```python
from build123d import *

# Parameters (mm, degrees)
FILLET2_SIZE = 0.5


with BuildPart() as part:
    # Sketch1 → Revolve1 (revolve)
    with BuildSketch(Plane.XY, mode=Mode.PRIVATE) as revolve1_sk:
        Polygon((0, 5), (3.5, 5), (6, 0), (2.75, 0), (2.75, 4), (0, 4), align=None)
    revolve(revolve1_sk.sketch.rotate(Axis((0, 0, 0), (0, 1, 0)), 90), axis=Axis((0, 0, 0), (0, 1, 0)))

    # Fillet1
    # a fillet whose section is not a circle: 0.5 mm, written as the material it takes off along each edge
    with BuildSketch(Plane(origin=(0, 5, 0), x_dir=(0, 0, -1), z_dir=(1, 0, 0))) as fillet1_piece_1:
        with BuildLine():
            add(Edge.make_bspline([(3.190983006, 0), (3.246118173, 0), (3.30125334, 0), (3.424221159, -0.01541979), (3.520097448, -0.074674596), (3.588882209, -0.177764417), (3.613539405, -0.22707881), (3.638196601, -0.276393202)], knots=[0, 0, 0, 0, 0, 0, 0.5, 0.5, 1, 1, 1, 1, 1, 1], degree=5))
            Line((3.638196601, -0.276393202), (3.5, 0))
            Line((3.5, 0), (3.190983006, 0))
        make_face()
    revolve(axis=Axis((0, 5, 0), (0, 1, 0)), mode=Mode.SUBTRACT)

    # Fillet2
    # a fillet whose section is not a circle: 0.5 mm, written as the material it takes off along each edge
    with BuildSketch(Plane(origin=(0, 0, 0), x_dir=(0, 0, -1), z_dir=(1, 0, 0))) as fillet2_piece_1:
        with BuildLine():
            add(Edge.make_bspline([(2.75 + FILLET2_SIZE, 0), (2.75 + FILLET2_SIZE * 0.831801948466, 0), (2.75 + FILLET2_SIZE * 0.663603896932, 0), (2.75 + FILLET2_SIZE * 0.292893218813, FILLET2_SIZE * 0.0716919198361), (2.75 + FILLET2_SIZE * 0.0716919198361, FILLET2_SIZE * 0.292893218813), (2.75, FILLET2_SIZE * 0.663603896932), (2.75, FILLET2_SIZE * 0.831801948466), (2.75, FILLET2_SIZE)], knots=[0, 0, 0, 0, 0, 0, 0.5, 0.5, 1, 1, 1, 1, 1, 1], degree=5))
            Line((2.75, FILLET2_SIZE), (2.75, 0))
            Line((2.75, 0), (2.75 + FILLET2_SIZE, 0))
        make_face()
    revolve(axis=Axis((0, 0, 0), (0, 1, 0)), mode=Mode.SUBTRACT)


solid = part.part
```
Input: part model. Units: mm. Frame: model coordinates. A direction names the side the tool comes from. Round coordinates to 2 decimals unless told otherwise and drop trailing zeros. Loops run counter-clockwise (first coordinate to the right, second up) from the corner with the lowest first, then second, coordinate; pieces in that order, holes last. Notation, with made-up numbers: M 70.5,36.25 L 104.5,36.25 A13 ccw 104.5,47.25 Z; hole C 41,83.5 d2. An arc over 180 degrees is marked long. Answer in a Markdown table with one row per item. Add a question column.
1. Section A-A (y = 1.8). Output: boundary loops of the cut face in (x, z), and give its area (3 significant figures).
2. Ray query, probe 1 along Z at (x, y) = (-2.25, 2.2); probe 2 along X at (y, z) = (2, 0.75); probe 3 along X at (y, z) = (1.5, 0). Return the intervals inside material, ascending.
3. Mould query, pull axis X, two halves, no side actions, for faces 3 (the face through (0, 5, 0)), 4 (the face through (-1.14, 4.43, -3.61)), 5 (the face through (0, 4, 0)). Classes: released by +X, released by -X, zero draft, split by the parting line, or undercut.
4. Contact query for flat-ended pins moving along their axis: pin 1 (3 mm diameter, centred on x = 3.5, y = 2, fed in from +Z); pin 2 (1 mm diameter, centred on y = 2, z = 0, fed in from -X); pin 3 (1 mm diameter, centred on y = 4, z = -0.5, fed in from -X). Output: stop coordinate, or through.
5. Set-up query: faces 1 (the face through (3, 0, -3)), 2 (the face through (2.685, 2.274, 0.596)). Return all of +Z, -Z, +X, -X, +Y, -Y with unobstructed straight access to the full face (end or side cutting, diameter ignored); none if empty.
6. Section B-B (y = 3.7). Output: boundary loops of the cut face in (x, z), and give its area (3 significant figures).
Values follow:
| question | item | result |
|---|---|---|
| 1 | outline | C 0,0 d10.2; hole C 0,0 d5.5 |
| 1 | area | 58.0 mm^2 |
| 2 | probe 1 | -4.35 to -1.58, 1.58 to 4.35 |
| 2 | probe 2 | -4.94 to -2.65, 2.65 to 4.94 |
| 2 | probe 3 | -5.25 to -2.75, 2.75 to 5.25 |
| 3 | face 3 | zero draft |
| 3 | face 4 | split by the parting line |
| 3 | face 5 | undercut |
| 4 | pin 1 | z = 4.97 |
| 4 | pin 2 | x = -5.25 |
| 4 | pin 3 | x = -4.23 |
| 5 | face 1 | +Z, -Z, +X, -X, -Y |
| 5 | face 2 | -Y |
| 6 | outline | C 0,0 d8.3; hole C 0,0 d5.5 |
| 6 | area | 30.3 mm^2 |
